CAD build for the part. Positions are in the model's coordinates, mm. Face numbers are marked on the shaded views. A direction names the side the tool comes from. Coordinates: 2 decimals unless noted, no trailing zeros. Order: outer loops, then holes, each group sorted by start corner. A loop starts at its lowest first (then second) coordinate and runs counter-clockwise, first axis right, second up. Notation, with made-up numbers: (-8.75, 87) - (13.25, 87) arc R34 cw to (13.25, 121) - close; hole circle Ø8 at (25, 79). An arc over 180 degrees is marked (long way). Use one line per item in the form item = value.
```python
from build123d import *

# Parameters (mm, degrees)
SKETCH1_R           = 5.922468873
SKETCH1_R_2         = 4.194729015
SKETCH1_R_3         = 0.79375
BOSS_EXTRUDE1_DEPTH = 6.35


with BuildPart() as part:
    # Sketch1 → Boss-Extrude1 (new body)
    # profile 1 of 3: a face of its own
    with BuildSketch(Plane(origin=(0, 0, 0), x_dir=(1, 0, 0), z_dir=(0, 1, 0))):
        Circle(SKETCH1_R)
        Circle(SKETCH1_R_2, mode=Mode.SUBTRACT)
    # profile 2 of 3: a face of its own
    with BuildSketch(Plane(origin=(0, 0, 0), x_dir=(1, 0, 0), z_dir=(0, 1, 0))):
        Circle(SKETCH1_R_2)
        with Locations(Location((0, 0, 0), (0, 0, 270))):
            Circle(SKETCH1_R_3, mode=Mode.SUBTRACT)
    # profile 3 of 3: a face of its own
    with BuildSketch(Plane(origin=(0, 0, 0), x_dir=(1, 0, 0), z_dir=(0, 1, 0))):
        with BuildLine():
            ThreePointArc((3.646669154, 25.4), (0, 29.046669154), (-3.646669154, 25.4))
            Line((-3.646669154, 25.4), (-3.646669154, 4.666630651))
            ThreePointArc((-3.646669154, 4.666630651), (0, 5.922468873), (3.646669154, 4.666630651))
            Line((3.646669154, 4.666630651), (3.646669154, 25.4))
        make_face()
        with Locations(Location((0, 20.32, 0), (0, 0, 270))):
            Circle(SKETCH1_R_3, mode=Mode.SUBTRACT)
        with Locations(Location((0, 25.4, 0), (0, 0, 270))):
            Circle(SKETCH1_R_3, mode=Mode.SUBTRACT)
    extrude(amount=BOSS_EXTRUDE1_DEPTH)


solid = part.part
```
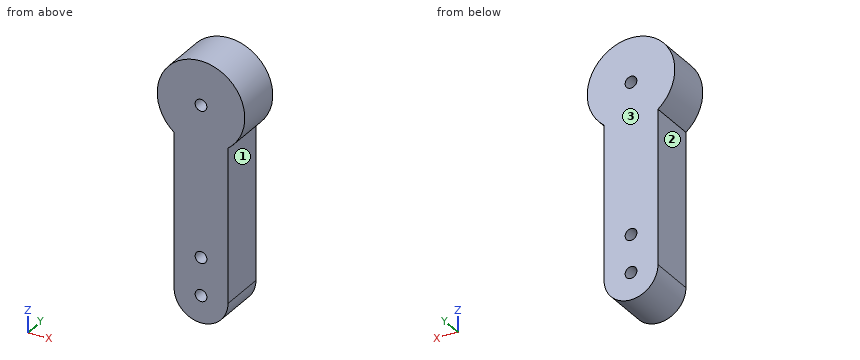
Item 1: Cut at C-C, the plane x = 0. Write the cut outline in (y, z).
Derived:
outline = (0, -29.05) - (6.35, -29.05) - (6.35, -26.19) - (0, -26.19) - close; (0, -24.61) - (6.35, -24.61) - (6.35, -21.11) - (0, -21.11) - close; (0, -19.53) - (6.35, -19.53) - (6.35, -0.79) - (0, -0.79) - close; (0, 0.79) - (6.35, 0.79) - (6.35, 5.92) - (0, 5.92) - close
Item 2: Cut at D-D, the plane z = 0. Write the cut outline in (x, y).
Derived:
outline = (-5.92, 0) - (-0.79, 0) - (-0.79, 6.35) - (-5.92, 6.35) - close; (0.79, 0) - (5.92, 0) - (5.92, 6.35) - (0.79, 6.35) - close
Item 3: Cut at A-A, the plane z = -20.32. Write the cut outline in (x, y), plus the area to 3 significant figures.
Derived:
outline = (-3.65, 0) - (-0.79, 0) - (-0.79, 6.35) - (-3.65, 6.35) - close; (0.79, 0) - (3.65, 0) - (3.65, 6.35) - (0.79, 6.35) - close
area = 36.2 mm²
Item 4: Drop flat-ended pins along their axis: pin 1 (3 mm diameter, centred on y = 3, z = -18, fed in from -X); pin 2 (1.4 mm diameter, centred on x = 0, z = -25.4, fed in from +Y); pin 3 (1 mm diameter, centred on x = 2, y = 2.5, fed in from -Z). Give the stop position or say it passes through.
Derived:
pin_1 = -3.65
pin_2 = through
pin_3 = -28.72
Item 5: Cut at B-B, the plane y = 1.25. Write the cut outline in (x, z), plus the area to 3 significant figures.
Derived:
outline = (-3.65, -25.4) arc R3.65 ccw to (3.65, -25.4) - (3.65, -4.67) arc R5.92 ccw (long way) to (-3.65, -4.67) - close; hole circle Ø1.59 at (0, -25.4); hole circle Ø1.59 at (0, -20.32); hole circle Ø1.59 at (0, 0)
area = 270 mm²
Item 6: Drill centre lines: line 1 (X direction, y = 1.5, z = -20.32); line 2 (X direction, y = 2.75, z = 0); line 3 (X direction, y = 3, z = -10.5). Where is each one in solid material? Low to high. Write a range as [from, to].
Derived:
line_1 = [-3.65, -0.79], [0.79, 3.65]
line_2 = [-5.92, -0.79], [0.79, 5.92]
line_3 = [-3.65, 3.65]
Item 7: 3-axis set-ups, long thin cutter, end or side, ignore diameter. For the marked faces 1, 2 and 3: which of +Z, -Z, +X, -X, +Y, -Y reach the whole face in a straight line?
Derived:
face_1 = -Z, +X, +Y, -Y
face_2 = -Z, -X, +Y, -Y
face_3 = +Z, -Z, +X, -X, +Y
